Verification items for this drawing (mm, ordinates from the low corner). Coordinates: 2 decimals unless noted, no trailing zeros. Order: outer loops, then holes, each group sorted by start corner. A loop starts at its lowest first (then second) coordinate and runs counter-clockwise, first axis right, second up. Notation, with made-up numbers: M 33.5,21.5 L 37.5,21.5 A21 cw 37.5,46.5 Z; hole C 74.25,80 d11. An arc over 180 degrees is marked long. Use CSV: the item, a comma, the result in double quotes. Start each with the question number.
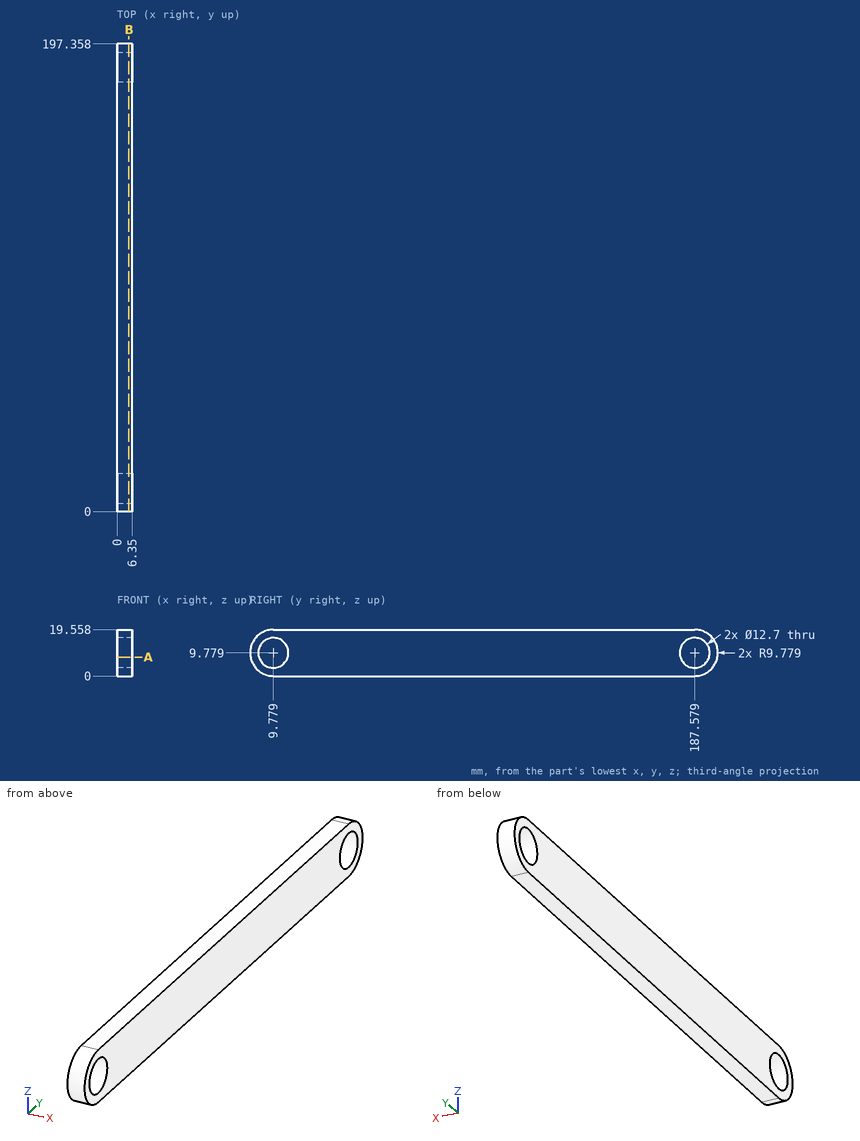
1) Section check A-A on z = 8. Record the boundary of the cut face in (x, y), then the cut area to 3 significant figures.
2) Section check B-B on x = 5. Record the boundary of the cut face in (y, z), then the cut area to 3 significant figures.
3) Material ranges on line 1 along Y through (x, z) = (2, 12.5); line 2 along Y through (x, z) = (5.75, 6.75); line 3 along Z through (x, y) = (3, 11.5), recorded low to high.
4) Gauge pin test, flat ends, axial feed: P1, Ø2, axis at x = 5.5, z = 17.5, coming from the +Y side; P2, Ø1.5, axis at x = 5.5, y = 119, coming from the -Z side; P3, Ø2, axis at x = 1.5, z = 5, coming from the +Y side; P4, Ø1.5, axis at x = 4, z = 12, coming from the -Y side. Record the tip position at first contact, or that the pin passes through.
Results are:
1,outline,"M 0,0.16 L 6.35,0.16 L 6.35,3.68 L 0,3.68 Z; M 0,15.87 L 6.35,15.87 L 6.35,181.48 L 0,181.48 Z; M 0,193.67 L 6.35,193.67 L 6.35,197.19 L 0,197.19 Z"
1,area,"1,100 mm²"
2,outline,"M 9.78,0 L 187.58,0 A9.78 ccw 187.58,19.56 L 9.78,19.56 A9.78 ccw Z; hole C 9.78,9.78 d12.7; hole C 187.58,9.78 d12.7"
2,area,"3,520 mm²"
3,line 1,"y = 0.39 to 4.04, 15.52 to 181.84, 193.32 to 196.97"
3,line 2,"y = 0.48 to 4.2, 15.36 to 182, 193.16 to 196.88"
3,line 3,"z = 0 to 3.67, 15.89 to 19.56"
4,P1,"stops at y = 194.68"
4,P2,"stops at z = 0"
4,P3,"stops at y = 196.6"
4,P4,"stops at y = 0.11"
